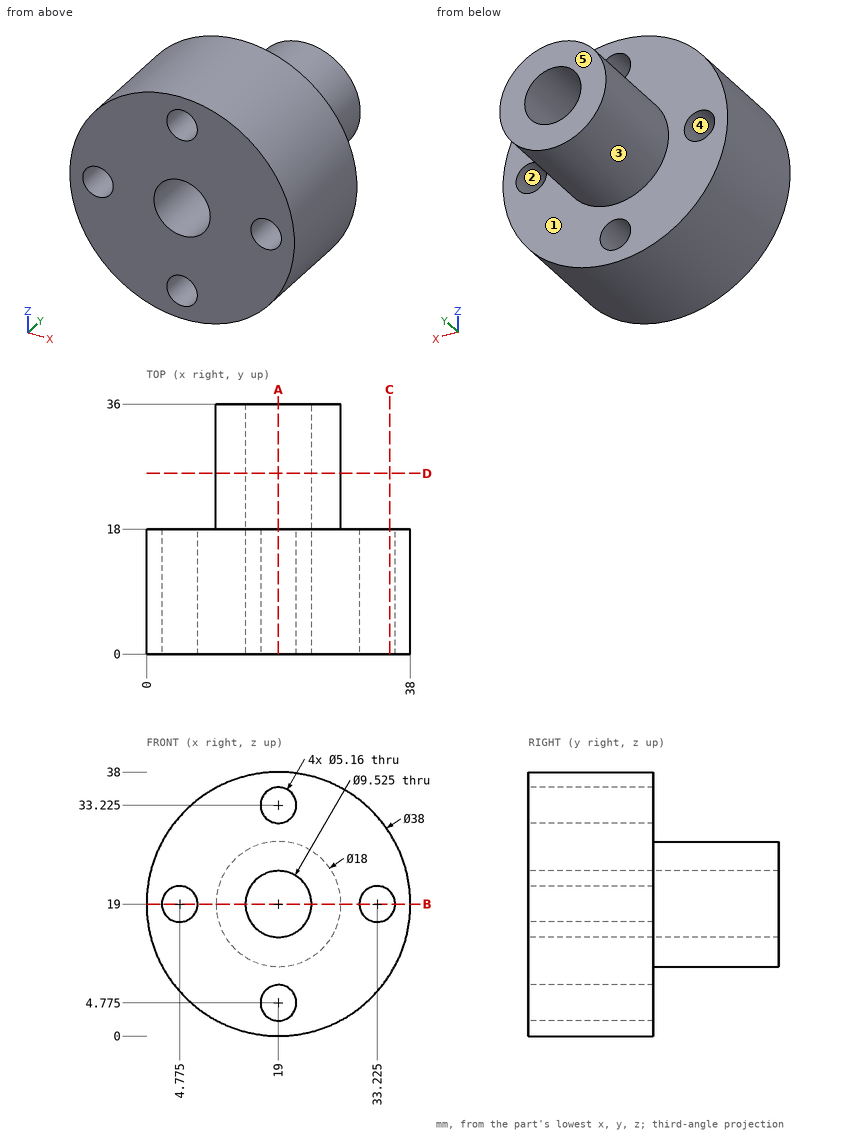
Verification items for this drawing (mm, ordinates from the low corner). A direction names the side the tool comes from. Give positions to 0.01 mm unless a question says otherwise; leave off trailing zeros. Write each loop counter-clockwise with the first axis right and the second up, starting at its lowest first coordinate (ties: lowest second). Pieces come first, ordered by that corner, then holes.
1) Section check D-D, the plane y = 26. Record the boundary of the cut face in (x, z) (1 decimal), and give its area (3 significant figures).
2) Gauge pin test, flat ends, axial feed: pin 1 (5 mm diameter, centred on x = 24.5, z = 12.5, fed in from -Y); pin 2 (8.5 mm diameter, centred on x = 19, z = 4.775, fed in from +Y); pin 3 (5 mm diameter, centred on y = 26.5, z = 18.5, fed in from +X); pin 4 (6 mm diameter, centred on x = 24.5, y = 6, fed in from +Z). Record the tip position at first contact, or that the pin passes through.
3) Access from +Z, -Z, +X, -X, +Y, -Y to the whole of each face (thin tool, end or side, straight path). Record for the marked faces 1 and 2.
4) Release check for a two-part mould opening along X. For the marked faces 3, 4 and 5 record: pulls with the +X half, pulls with the -X half, needs draft (parallel to the pull), parting line crosses it, or undercut.
5) Section check B-B, the plane z = 19. Record the boundary of the cut face in (x, y) (1 decimal), and give its area (3 significant figures).
6) Section check C-C, the plane x = 35. Record the boundary of the cut face in (y, z).
7) Section check A-A, the plane x = 19. Record the boundary of the cut face in (y, z) (1 decimal).
8) Material ranges on L1, parallel to Z at x = 19, y = 7.25 (1 decimal); L2, parallel to Z at x = 17, y = 12; L3, parallel to Y at x = 8, z = 16.5, recorded low to high.
Computed:
1. outline: circle Ø18 at (19, 19); hole circle Ø9.5 at (19, 19)
1. area: 183 mm2
2. pin 1: stops at y = 0
2. pin 2: stops at y = 18
2. pin 3: stops at x = 28
2. pin 4: stops at z = 37.83
3. face 1: +Y
3. face 2: +Y, -Y
4. face 3: parting line crosses it
4. face 4: undercut
4. face 5: needs draft
5. outline: (0, 0) - (2.2, 0) - (2.2, 18) - (0, 18) - close; (7.4, 0) - (14.2, 0) - (14.2, 36) - (10, 36) - (10, 18) - (7.4, 18) - close; (23.8, 0) - (30.6, 0) - (30.6, 18) - (28, 18) - (28, 36) - (23.8, 36) - close; (35.8, 0) - (38, 0) - (38, 18) - (35.8, 18) - close
5. area: 479 mm2
6. outline: (0, 8.75) - (18, 8.75) - (18, 17.13) - (0, 17.13) - close; (0, 20.87) - (18, 20.87) - (18, 29.25) - (0, 29.25) - close
7. outline: (0, 0) - (18, 0) - (18, 2.2) - (0, 2.2) - close; (0, 7.4) - (18, 7.4) - (18, 10) - (36, 10) - (36, 14.2) - (0, 14.2) - close; (0, 23.8) - (36, 23.8) - (36, 28) - (18, 28) - (18, 30.6) - (0, 30.6) - close; (0, 35.8) - (18, 35.8) - (18, 38) - (0, 38) - close
8. L1: z = 0 to 2.2, 7.4 to 14.2, 23.8 to 30.6, 35.8 to 38
8. L2: z = 0.11 to 3.15, 6.4 to 14.68, 23.32 to 31.6, 34.85 to 37.89
8. L3: y = 0 to 18
